```python
from build123d import *

# Parameters (mm, degrees)
SKETCH1_W           = 13.7795
SKETCH1_H           = 117.97300002
BOSS_EXTRUDE1_DEPTH = 3.175
SKETCH5_W           = 13.7795
SKETCH5_H           = 9.525
BOSS_EXTRUDE2_DEPTH = 6.35
SKETCH4_R           = 1.399999994
CUT_EXTRUDE1_DEPTH  = 118.97300002
BOSS_EXTRUDE3_DEPTH = 13.7795
FILLET1_R           = 3.175


with BuildPart() as part:
    # Sketch1 → Boss-Extrude1 (new body)
    with BuildSketch(Plane(origin=(0, 0, 0), x_dir=(1, 0, 0), z_dir=(0, 1, 0))):
        Rectangle(SKETCH1_W, SKETCH1_H)
    extrude(amount=BOSS_EXTRUDE1_DEPTH)

    # Sketch5 → Boss-Extrude2 (add)
    with BuildSketch(Plane.XY.offset(58.98650001)):
        with Locations((0, 7.9375)):
            Rectangle(SKETCH5_W, SKETCH5_H)
    boss_extrude2 = extrude(amount=-BOSS_EXTRUDE2_DEPTH)

    # Mirror1: Boss-Extrude2 across plane
    add(boss_extrude2.mirror(Plane.XY))

    # Sketch4 → Cut-Extrude1 (cut, through all)
    with BuildSketch(Plane.XY.offset(58.98650001)):
        with Locations((0, 6.35)):
            Circle(SKETCH4_R)
    extrude(amount=-CUT_EXTRUDE1_DEPTH, mode=Mode.SUBTRACT)

    # Sketch6 → Boss-Extrude3 (add)
    with BuildSketch(Plane.ZY.offset(6.88975)):
        Polygon((-11.36150001, 6.985), (-5.01150001, 6.985), (5.456388958, 3.175), (-21.829388978, 3.175), align=None)
    extrude(amount=-BOSS_EXTRUDE3_DEPTH)

    # Fillet1
    fillet1_edges = [part.edges().sort_by_distance(p)[0] for p in [
        (0, 3.175, -21.829388978),
        (0, 6.985, -11.36150001),
        (0, 6.985, -5.01150001),
        (0, 3.175, 5.456388958),
    ]]
    fillet(fillet1_edges, radius=FILLET1_R)


solid = part.part
```
Geometry: final body of the model. Coordinates: model frame, mm. A direction names the side the tool comes from. Round coordinates to 2 decimals unless told otherwise and drop trailing zeros. Order: outer loops, then holes, each group sorted by start corner. A loop starts at its lowest first (then second) coordinate and runs counter-clockwise, first axis right, second up. Notation, with made-up numbers: (15, 31) - (59, 31) arc R21 cw to (59, 61) - close; hole circle Ø4 at (-5.5, 15). An arc over 180 degrees is marked (long way). Write item = value, one per line. Start each with the question number.
Q1. Pin query (flat end, axial travel): pin 1 (2.5 mm diameter, centred on x = 0, z = -8, fed in from +Y) (3 decimals); pin 2 (6 mm diameter, centred on x = 1, z = 14, fed in from +Y) (3 decimals). Return the tip coordinate at first contact, or that it passes through.
Q2. Cut plane A-A on y = 10. Return the cut outline in (x, z).
Q3. Pull-direction query (X, two-part tool) for faces 4 (the flat face through (-6.89, 3, -5)), 5 (the flat face through (6.89, 3, -5)), 6 (the flat face through (-0.096, 5.104, 0.157)), 7 (the cylindrical face through (-0.303, 4.983, -55.767)); classes: +X half, -X half, draft (parallel to the pull), parting line (faces both ways), or undercut.
Q4. Cut plane B-B on x = 0. Give the number of separate pieces and of enclosed holes in the cut face, and give its area (3 significant figures).
Q5. Ray query, line 1 (Z direction, x = -5.5, y = 9.25); line 2 (Y direction, x = 0, z = 56.5); line 3 (Y direction, x = 1.75, z = 9.5) (3 decimals). Return the intervals inside material, ascending. Write a range as from..to.
Q6. Access query for faces 1 (the cylindrical face through (-0.303, 4.983, 55.856)), 2 (the flat face through (0, 3.175, -38)), 3 (the flat face through (0, 8, -58.987)). Directions: +Z, -Z, +X, -X, +Y, -Y. A direction counts if a zero-diameter tool reaches every point of the face in a straight line with its end or side. Return the directions, or none.
Q7. Cut plane D-D on z = 16.5. Return the cut outline in (x, y) (3 decimals), and give its area (4 significant figures).
Outcome:
q1.pin_1 = 6.985
q1.pin_2 = 3.175
q2.outline = (-6.89, -58.99) - (6.89, -58.99) - (6.89, -52.64) - (-6.89, -52.64) - close; (-6.89, 52.64) - (6.89, 52.64) - (6.89, 58.99) - (-6.89, 58.99) - close
q3.face_4 = -X half
q3.face_5 = +X half
q3.face_6 = draft
q3.face_7 = undercut
q4.separate_pieces = 3
q4.enclosed_holes = 0
q4.area = 524 mm^2
q5.line_1 = -58.99..-52.64, 52.64..58.99
q5.line_2 = 0..4.95, 7.75..12.7
q5.line_3 = 0..3.175
q6.face_1 = +Z
q6.face_2 = +X, -X, +Y
q6.face_3 = -Z, +X, -X, +Y, -Y
q7.outline = (-6.89, 0) - (6.89, 0) - (6.89, 3.175) - (-6.89, 3.175) - close
q7.area = 43.75 mm^2
